Here's how the part is built. I have some questions about the finished solid (model axes, mm). Face numbers are marked on the shaded views. A direction names the side the tool comes from. Coordinates: 2 decimals unless noted, no trailing zeros. Write each loop counter-clockwise with the first axis right and the second up, starting at its lowest first coordinate (ties: lowest second). Pieces come first, ordered by that corner, then holes. Notation, with made-up numbers: (51.5, 25) - (75.5, 25) arc R22 ccw to (75.5, 47) - close; hole circle Ø9 at (7, -35). An arc over 180 degrees is marked (long way). Answer in a Markdown table with one row per item. Add a question column.
Item 1: Which directions (+Z, -Z, +X, -X, +Y, -Y) give clear straight access to the entire face, cutting with the end or side of a thin tool? Please do the marked faces 4 and 5.
Item 2: We'd pull the mould along Y, two halves only. Please class the marked faces 1, 2 and 3: +Y half, -Y half, draft (parallel to the pull), parting line (faces both ways), or undercut.
Item 3: Imagine slicing it at A-A (z = 23). Please give me the cut outline in (x, y), plus the area to 3 significant figures.
Item 4: Imagine slicing it at C-C (y = -2.5). Please give me the cut outline in (x, z).
Item 5: Imagine slicing it at D-D (x = 2). Please give me the cut outline in (y, z), plus the area to 3 significant figures.
Item 6: If I drill on probe 1 along Z at (x, y) = (0, -0.65); probe 2 along X at (y, z) = (0.95, 35); probe 3 along Y at (x, z) = (0.5, 6), over which ranges is the centre line in solid material (lowest first)? Write a range as from..to.
Item 7: Imagine slicing it at B-B (z = 28.5). Please give me the cut outline in (x, y).
Item 8: I'm going to push flat-ended pins straight in: pin 1 (1 mm diameter, centred on x = -3, z = 17.5, fed in from -Y); pin 2 (0.7 mm diameter, centred on x = 3, y = -0.5, fed in from +Z); pin 3 (1 mm diameter, centred on x = 3, z = 16.5, fed in from +Y); pin 4 (3.5 mm diameter, centred on y = 0, z = 13, fed in from -X). Where does each tip first touch, or does it pass through?
from build123d import *

# Parameters (mm, degrees)
EXTRUDE_1_DEPTH      = 30
EXTRUDE_2_DEPTH      = 1
SKETCH_3_W           = 26
SKETCH_3_H           = 2.5
CUT_EXTRUDE_1_DEPTH  = 6.928203
SKETCH_7_R           = 1
EXTRUDE_3_DEPTH      = 1.5
EXTRUDE_3_DEPTH_BACK = 1.5


with BuildPart() as part:
    # 스케치1 → 보스-돌출1 (new body)
    with BuildSketch(Plane.XY):
        Polygon((0, 4), (-3.464101615, 2), (-3.464101615, -2), (0, -4), (3.464101615, -2), (3.464101615, 2), align=None)
        Polygon((0, 3), (-2.598076211, 1.5), (-2.598076211, -1.5), (0, -3), (2.598076211, -1.5), (2.598076211, 1.5), align=None, mode=Mode.SUBTRACT)
    extrude(amount=EXTRUDE_1_DEPTH)

    # 스케치4 → 보스-돌출2 (add)
    with BuildSketch(Plane.XY.offset(30)):
        Polygon((0, 4), (-3.464101615, 2), (-3.464101615, -2), (0, -4), (3.464101615, -2), (3.464101615, 2), align=None)
    extrude(amount=EXTRUDE_2_DEPTH)

    # 스케치3 → 컷-돌출1 (cut)
    with BuildSketch(Plane(origin=(3.464101615, 0, 0), x_dir=(0, 0, -1), z_dir=(1, 0, 0))):
        with Locations((-15, 0)):
            Rectangle(SKETCH_3_W, SKETCH_3_H)
    extrude(amount=-CUT_EXTRUDE_1_DEPTH, mode=Mode.SUBTRACT)

    # 스케치7 → 보스-돌출3 (add, two sides)
    with BuildSketch(Plane(origin=(0, 0, 0), x_dir=(1, 0, 0), z_dir=(0, 1, 0))) as extrude_3_sk:
        with BuildLine():
            Line((3.464101615, -31), (-3.464101615, -31))
            Line((-3.464101615, -31), (-3.464101615, -35))
            ThreePointArc((-3.464101615, -35), (0, -38.464101615), (3.464101615, -35))
            Line((3.464101615, -35), (3.464101615, -31))
        make_face()
        with Locations((0, -35)):
            Circle(SKETCH_7_R, mode=Mode.SUBTRACT)
    extrude(amount=EXTRUDE_3_DEPTH)
    extrude(extrude_3_sk.sketch, amount=-EXTRUDE_3_DEPTH_BACK)


solid = part.part
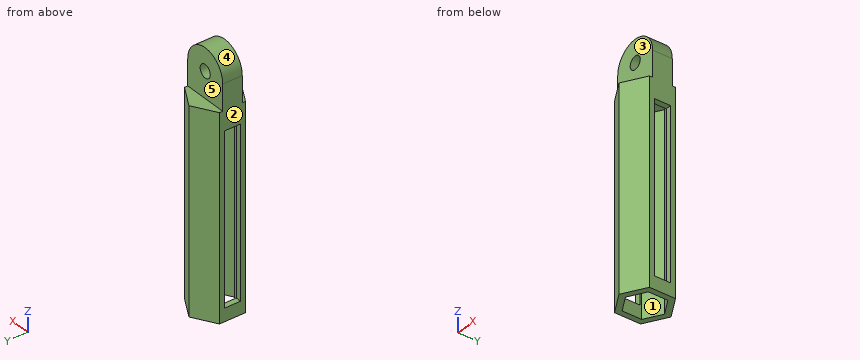
Here are the results:
| question | item | result |
|---|---|---|
| 1 | face 4 | +Z, +Y, -Y |
| 1 | face 5 | +Z, +X, -X, +Y |
| 2 | face 1 | undercut |
| 2 | face 2 | draft |
| 2 | face 3 | -Y half |
| 3 | outline | (-3.46, -2) - (0, -4) - (3.46, -2) - (3.46, -1.25) - (2.6, -1.25) - (2.6, -1.5) - (0, -3) - (-2.6, -1.5) - (-2.6, -1.25) - (-3.46, -1.25) - close; (-3.46, 1.25) - (-2.6, 1.25) - (-2.6, 1.5) - (0, 3) - (2.6, 1.5) - (2.6, 1.25) - (3.46, 1.25) - (3.46, 2) - (0, 4) - (-3.46, 2) - close |
| 3 | area | 13.9 mm2 |
| 4 | outline | (-2.6, 0) - (-0.87, 0) - (-0.87, 30) - (0.87, 30) - (0.87, 0) - (2.6, 0) - (2.6, 31) - (-2.6, 31) - close |
| 5 | outline | (-2.85, 0) - (-1.85, 0) - (-1.85, 30) - (1.85, 30) - (1.85, 0) - (2.85, 0) - (2.85, 31) - (1.5, 31) - (1.5, 37.83) - (-1.5, 37.83) - (-1.5, 31) - (-2.85, 31) - close |
| 5 | area | 86.2 mm2 |
| 6 | probe 1 | z = 30..34, 36..38.46 |
| 6 | probe 2 | x = -3.46..-1, 1..3.46 |
| 6 | probe 3 | y = -3.71..-2.71, 2.71..3.71 |
| 7 | outline | (-3.46, -2) - (0, -4) - (3.46, -2) - (3.46, 2) - (0, 4) - (-3.46, 2) - close; hole (-2.6, -1.5) - (0, -3) - (2.6, -1.5) - (2.6, 1.5) - (0, 3) - (-2.6, 1.5) - close |
| 8 | pin 1 | stops at y = -2.56 |
| 8 | pin 2 | stops at z = 37.23 |
| 8 | pin 3 | stops at y = 2.56 |
| 8 | pin 4 | stops at x = -3.46 |
